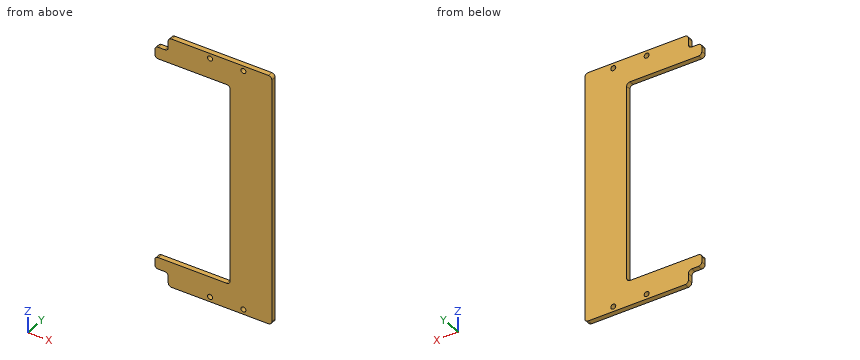
```python
from build123d import *

# Parameters (mm, degrees)
EXTRUDE_1_DEPTH     = 3
SKETCH_2_W          = 8
SKETCH_2_H          = 8
CUT_EXTRUDE_1_DEPTH = 10
SKETCH_3_R          = 1.5
CUT_EXTRUDE_2_DEPTH = 10
FILLET_1_R          = 2


with BuildPart() as part:
    # 草图1 → 凸台-拉伸1 (new body)
    with BuildSketch(Plane(origin=(0, 0, 0), x_dir=(1, 0, 0), z_dir=(0, 1, 0))):
        Polygon((0, 0), (70, 0), (70, 150), (0, 150), (0, 135), (45, 135), (45, 15), (0, 15), align=None)
    extrude(amount=EXTRUDE_1_DEPTH)

    # 草图2 → 切除-拉伸1 (cut)
    with BuildSketch(Plane(origin=(0, 3, 0), x_dir=(1, 0, 0), z_dir=(0, 1, 0))):
        with Locations((4, 4)):
            Rectangle(SKETCH_2_W, SKETCH_2_H)
        with Locations((4, 146)):
            Rectangle(SKETCH_2_W, SKETCH_2_H)
    extrude(amount=-CUT_EXTRUDE_1_DEPTH, mode=Mode.SUBTRACT)

    # 草图3 → 切除-拉伸2 (cut)
    with BuildSketch(Plane(origin=(0, 3, 0), x_dir=(1, 0, 0), z_dir=(0, 1, 0))):
        with Locations(Location((33, 3, 0), (0, 0, 270))):
            Circle(SKETCH_3_R)
        with Locations(Location((53, 3, 0), (0, 0, 270))):
            Circle(SKETCH_3_R)
        with Locations(Location((53, 147, 0), (0, 0, 270))):
            Circle(SKETCH_3_R)
        with Locations(Location((33, 147, 0), (0, 0, 270))):
            Circle(SKETCH_3_R)
    extrude(amount=-CUT_EXTRUDE_2_DEPTH, mode=Mode.SUBTRACT)

    # 圆角1
    fillet_1_edges = [part.edges().sort_by_distance(p)[0] for p in [
        (0, 1.5, -15),
        (45, 1.5, -15),
        (45, 1.5, -135),
        (0, 1.5, -135),
        (70, 1.5, -150),
        (70, 1.5, 0),
        (8, 1.5, 0),
        (0, 1.5, -8),
        (8, 1.5, -8),
        (0, 1.5, -142),
        (8, 1.5, -150),
        (8, 1.5, -142),
    ]]
    fillet(fillet_1_edges, radius=FILLET_1_R)


solid = part.part
```
Model file for the job. Use its own axes, mm. Coordinates: 2 decimals unless noted, no trailing zeros. Loops run counter-clockwise (first coordinate to the right, second up) from the corner with the lowest first, then second, coordinate; pieces in that order, holes last. Notation, with made-up numbers: (28.5, -21) - (75.5, -21) arc R25 cw to (75.5, 15) - close; hole circle Ø3 at (0, 35.5). An arc over 180 degrees is marked (long way). Write item = value, one per line. Start each with the question number.
Item 1: Saw through at A-A, the plane x = 4. List the corners of the cut face in (y, z).
Item 2: Saw through at B-B, the plane x = 33. List the corners of the cut face in (y, z), then the cut area to 3 significant figures.
Item 3: Saw through at D-D, the plane x = 53. List the corners of the cut face in (y, z), then the cut area to 3 significant figures.
Item 4: Wall check: probe 1 along X at (y, z) = (1.05, -147); probe 2 along Z at (x, y) = (39, 0.95); probe 3 along X at (y, z) = (2.55, -65). Give the ranges that are in metal, low to high. Write a range as [from, to].
Item 5: Drop flat-ended pins along their axis: pin 1 Ø2.5 at (x, z) = (33, -3) entering from -Y; pin 2 Ø0.9 at (x, y) = (5, 2) entering from -Z; pin 3 Ø0.9 at (x, y) = (3, 1) entering from +Z. Give the stop position or say it passes through.
Item 6: Saw through at C-C, the plane y = 1.8. List the corners of the cut face in (x, z).
Answers:
q1.outline = (0, -142) - (3, -142) - (3, -135) - (0, -135) - close; (0, -15) - (3, -15) - (3, -8) - (0, -8) - close
q2.outline = (0, -150) - (3, -150) - (3, -148.5) - (0, -148.5) - close; (0, -145.5) - (3, -145.5) - (3, -135) - (0, -135) - close; (0, -15) - (3, -15) - (3, -4.5) - (0, -4.5) - close; (0, -1.5) - (3, -1.5) - (3, 0) - (0, 0) - close
q2.area = 72.0 mm2
q3.outline = (0, -150) - (3, -150) - (3, -148.5) - (0, -148.5) - close; (0, -145.5) - (3, -145.5) - (3, -4.5) - (0, -4.5) - close; (0, -1.5) - (3, -1.5) - (3, 0) - (0, 0) - close
q3.area = 432 mm2
q4.probe_1 = [8, 31.5], [34.5, 51.5], [54.5, 70]
q4.probe_2 = [-150, -135], [-15, 0]
q4.probe_3 = [45, 70]
q5.pin_1 = through
q5.pin_2 = -142
q5.pin_3 = -8
q6.outline = (0, -140) arc R2 ccw to (2, -142) - (6, -142) arc R2 cw to (8, -144) - (8, -148) arc R2 ccw to (10, -150) - (68, -150) arc R2 ccw to (70, -148) - (70, -2) arc R2 ccw to (68, 0) - (10, 0) arc R2 ccw to (8, -2) - (8, -6) arc R2 cw to (6, -8) - (2, -8) arc R2 ccw to (0, -10) - (0, -13) arc R2 ccw to (2, -15) - (43, -15) arc R2 cw to (45, -17) - (45, -133) arc R2 cw to (43, -135) - (2, -135) arc R2 ccw to (0, -137) - close; hole circle Ø3 at (33, -147); hole circle Ø3 at (33, -3); hole circle Ø3 at (53, -147); hole circle Ø3 at (53, -3)
